Here's how the part is built. I have some questions about the finished solid (model axes, mm). Face numbers are marked on the shaded views. A direction names the side the tool comes from. Coordinates: 2 decimals unless noted, no trailing zeros. Write each loop counter-clockwise with the first axis right and the second up, starting at its lowest first coordinate (ties: lowest second). Pieces come first, ordered by that corner, then holes. Notation, with made-up numbers: M -26.5,27 L 28.5,27 A20 ccw 28.5,53 Z; hole C 65,-7.75 d5. An arc over 180 degrees is marked long. Write each question's results on one line, items separated by ' | '. Start each with the question number.
from build123d import *

# Parameters (mm, degrees)
SKETCH_1_W                     = 112
SKETCH_1_H                     = 112
SKETCH_1_W_2                   = 106
SKETCH_1_H_2                   = 106
EXTRUDE_1_DEPTH                = 45
SKETCH_3_W                     = 112
SKETCH_3_H                     = 112
EXTRUDE_2_DEPTH                = 6
SKETCH_4_R                     = 28.5
CUT_EXTRUDE_2_DEPTH            = 2
SKETCH_5_R                     = 2.05
CUT_EXTRUDE_3_DEPTH            = 3
SKETCH_6_R                     = 17
CUT_EXTRUDE_4_DEPTH            = 6
EXTRUDE_3_DEPTH                = 9
FILLET_1_R                     = 5
SKETCH_8_W                     = 85
SKETCH_8_H                     = 15
CUT_EXTRUDE_5_DEPTH            = 5
SKETCH_9_W                     = 25
SKETCH_9_H                     = 15
CUT_EXTRUDE_6_DEPTH            = 5
SKETCH_10_R                    = 2.05
CUT_EXTRUDE_7_DEPTH            = 5
FILLET_5_R                     = 5
HOLE_WIZARD_M3_5_2_D           = 3.9
HOLE_WIZARD_M3_5_2_CSINK_D     = 7.7
HOLE_WIZARD_M3_5_2_CSINK_ANGLE = 90
FILLET_START                   = 9
FILLET_7_DEPTH                 = 31
FILLET_START_2                 = 40
FILLET_7_2_DEPTH               = 5


with BuildPart() as part:
    # 草图1 → 凸台-拉伸1 (new body)
    with BuildSketch(Plane(origin=(0, 0, 0), x_dir=(1, 0, 0), z_dir=(0, 1, 0))):
        Rectangle(SKETCH_1_W, SKETCH_1_H)
        Rectangle(SKETCH_1_W_2, SKETCH_1_H_2, mode=Mode.SUBTRACT)
    extrude(amount=EXTRUDE_1_DEPTH)

    # 草图3 → 凸台-拉伸2 (add)
    with BuildSketch(Plane.XZ):
        Rectangle(SKETCH_3_W, SKETCH_3_H)
    extrude(amount=EXTRUDE_2_DEPTH)

    # 草图4 → 切除-拉伸2 (cut)
    with BuildSketch(Plane.XZ.offset(6)):
        with Locations(Location((0, 0, 0), (0, 0, 270))):
            Circle(SKETCH_4_R)
    extrude(amount=-CUT_EXTRUDE_2_DEPTH, mode=Mode.SUBTRACT)

    # 草图5 → 切除-拉伸3 (cut)
    with BuildSketch(Plane(origin=(0, -4, 0), x_dir=(-1, 0, 0), z_dir=(0, -1, 0))):
        with Locations(Location((0, -22.5, 0), (0, 0, 90))):
            Circle(SKETCH_5_R)
        with Locations(Location((-22.5, 0, 0), (0, 0, 90))):
            Circle(SKETCH_5_R)
        with Locations(Location((22.5, 0, 0), (0, 0, 90))):
            Circle(SKETCH_5_R)
        with Locations(Location((0, 22.5, 0), (0, 0, 90))):
            Circle(SKETCH_5_R)
    extrude(amount=-CUT_EXTRUDE_3_DEPTH, mode=Mode.SUBTRACT)

    # 草图6 → 切除-拉伸4 (cut)
    with BuildSketch(Plane.XZ.offset(4)):
        with Locations(Location((0, 0, 0), (0, 0, 270))):
            Circle(SKETCH_6_R)
    extrude(amount=-CUT_EXTRUDE_4_DEPTH, mode=Mode.SUBTRACT)

    # 草图7 → 凸台-拉伸3 (add)
    with BuildSketch(Plane(origin=(0, 0, 0), x_dir=(1, 0, 0), z_dir=(0, 1, 0))):
        with BuildLine():
            Line((-45, 37), (-53, 37))
            Line((-53, 37), (-53, 53))
            Line((-53, 53), (-37, 53))
            Line((-37, 53), (-37, 45))
            ThreePointArc((-37, 45), (-39.343145751, 39.343145751), (-45, 37))
        make_face()
        with BuildLine():
            Line((-45, -37), (-53, -37))
            Line((-53, -37), (-53, -53))
            Line((-53, -53), (-37, -53))
            Line((-37, -53), (-37, -45))
            ThreePointArc((-37, -45), (-39.343145751, -39.343145751), (-45, -37))
        make_face()
        with BuildLine():
            Line((45, -39), (53, -39))
            Line((53, -39), (53, -53))
            Line((53, -53), (39, -53))
            Line((39, -53), (39, -45))
            ThreePointArc((39, -45), (41, -41), (45, -39))
        make_face()
        with BuildLine():
            Line((45, 37), (53, 37))
            Line((53, 37), (53, 53))
            Line((53, 53), (37, 53))
            Line((37, 53), (37, 45))
            ThreePointArc((37, 45), (39.343145751, 39.343145751), (45, 37))
        make_face()
    extrude(amount=EXTRUDE_3_DEPTH)

    # 圆角1
    fillet_1_edges = [part.edges().sort_by_distance(p)[0] for p in [
        (56, 19.5, 56),
        (-56, 19.5, 56),
        (-56, 19.5, -56),
        (56, 19.5, -56),
    ]]
    fillet(fillet_1_edges, radius=FILLET_1_R)

    # 草图8 → 切除-拉伸5 (cut)
    with BuildSketch(Plane.ZY.offset(56)):
        with Locations((0, 34.5)):
            Rectangle(SKETCH_8_W, SKETCH_8_H)
    extrude(amount=-CUT_EXTRUDE_5_DEPTH, mode=Mode.SUBTRACT)

    # 草图9 → 切除-拉伸6 (cut)
    with BuildSketch(Plane.XY.offset(56)):
        with Locations((18.5, 34.5)):
            Rectangle(SKETCH_9_W, SKETCH_9_H)
    extrude(amount=-CUT_EXTRUDE_6_DEPTH, mode=Mode.SUBTRACT)

    # 草图10 → 切除-拉伸7 (cut)
    with BuildSketch(Plane(origin=(0, 45, 0), x_dir=(1, 0, 0), z_dir=(0, 1, 0))):
        with Locations((52.035533906, -52.035533906)):
            Circle(SKETCH_10_R)
        with Locations((-52.035533906, -52.035533906)):
            Circle(SKETCH_10_R)
        with Locations((-52.035533906, 52.035533906)):
            Circle(SKETCH_10_R)
        with Locations((52.035533906, 52.035533906)):
            Circle(SKETCH_10_R)
    extrude(amount=-CUT_EXTRUDE_7_DEPTH, mode=Mode.SUBTRACT)

    # 圆角5
    fillet_5_edges = [part.edges().sort_by_distance(p)[0] for p in [
        (56, -6, 0),
        (-56, -6, 0),
        (0, -6, -56),
        (0, -6, 56),
        (-54.535533906, -6, 54.535533906),
        (-54.535533906, -6, -54.535533906),
        (54.535533906, -6, -54.535533906),
        (54.535533906, -6, 54.535533906),
    ]]
    fillet(fillet_5_edges, radius=FILLET_5_R)

    # M3.5 十字槽半沉头木螺钉的锥形沉头孔2 (through all)
    with Locations(Plane(origin=(0, -6, 0), x_dir=(-1, 0, 0), z_dir=(0, -1, 0))):
        with Locations((0, 0), (45, -45), (-45, 45), (-45, -45), (45, 45)):
            CounterSinkHole(HOLE_WIZARD_M3_5_2_D / 2, HOLE_WIZARD_M3_5_2_CSINK_D / 2, counter_sink_angle=HOLE_WIZARD_M3_5_2_CSINK_ANGLE)

    # 圆角7: read off the stored shape, not the designer's step
    # 圆角7 outline → 圆角7 (add)
    with BuildSketch(Plane(origin=(0, 0, 0), x_dir=(1, 0, 0), z_dir=(0, 1, 0)).offset(FILLET_START)):
        with BuildLine():
            Line((53, -53), (53, -43))
            ThreePointArc((53, -43), (50.071067812, -50.071067812), (43, -53))
            Line((43, -53), (53, -53))
        make_face()
        with BuildLine():
            ThreePointArc((43, 53), (50.071067812, 50.071067812), (53, 43))
            Line((53, 43), (53, 53))
            Line((53, 53), (43, 53))
        make_face()
        with BuildLine():
            ThreePointArc((-43, -53), (-50.071067812, -50.071067812), (-53, -43))
            Line((-53, -43), (-53, -53))
            Line((-53, -53), (-43, -53))
        make_face()
        with BuildLine():
            ThreePointArc((-53, 43), (-50.071067812, 50.071067812), (-43, 53))
            Line((-43, 53), (-53, 53))
            Line((-53, 53), (-53, 43))
        make_face()
    extrude(amount=FILLET_7_DEPTH)

    # Fillet 7 2 outline → Fillet 7 2 (add)
    with BuildSketch(Plane(origin=(0, 0, 0), x_dir=(1, 0, 0), z_dir=(0, 1, 0)).offset(FILLET_START_2)):
        with BuildLine():
            ThreePointArc((50.22658251, -53), (50.585965005, -50.585965005), (53, -50.22658251))
            Line((53, -50.22658251), (53, -43))
            ThreePointArc((53, -43), (50.071067812, -50.071067812), (43, -53))
            Line((43, -53), (50.22658251, -53))
        make_face()
        with BuildLine():
            ThreePointArc((43, 53), (50.071067812, 50.071067812), (53, 43))
            Line((53, 43), (53, 50.22658251))
            ThreePointArc((53, 50.22658251), (50.585965005, 50.585965005), (50.22658251, 53))
            Line((50.22658251, 53), (43, 53))
        make_face()
        with BuildLine():
            Line((-50.22658251, -53), (-43, -53))
            ThreePointArc((-43, -53), (-50.071067812, -50.071067812), (-53, -43))
            Line((-53, -43), (-53, -50.22658251))
            ThreePointArc((-53, -50.22658251), (-50.585965005, -50.585965005), (-50.22658251, -53))
        make_face()
        with BuildLine():
            ThreePointArc((-53, 43), (-50.071067812, 50.071067812), (-43, 53))
            Line((-43, 53), (-50.22658251, 53))
            ThreePointArc((-50.22658251, 53), (-50.585965005, 50.585965005), (-53, 50.22658251))
            Line((-53, 50.22658251), (-53, 43))
        make_face()
    extrude(amount=FILLET_7_2_DEPTH)


solid = part.part
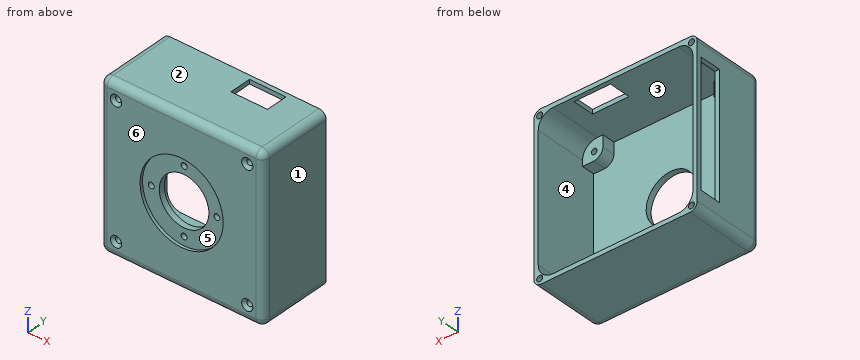
1) Please list where these lines run through material, in increasing order: line 1 (Z direction, x = 45, y = -1); line 2 (X direction, y = 3, z = -45); line 3 (Z direction, x = 45, y = 1.75). Write a range as [from, to].
2) For the marked faces 4, 5 and 6, which set-ups out of +Z, -Z, +X, -X, +Y, -Y let a thin tool reach every point of the face, with its end or its side?
3) For pin 1 Ø4.5 at (x, z) = (0, 22.5) entering from -Y; pin 2 Ø3.5 at (x, z) = (52.04, 52.04) entering from +Y; pin 3 Ø3.5 at (x, z) = (-45, 45) entering from +Y; pin 4 Ø6 at (x, z) = (45, 45) entering from -Y, each with a flat end and sliding along its axis, tell me the tip position at first contact or that it passes through.
4) I want a section at A-A, the plane x = 0. Write out the boundary of the cut face in (y, z).
5) I want a section at D-D, the plane y = 24. Write out the boundary of the cut face in (x, z), then the cut area to 3 significant figures.
6) We'd pull the mould along Z, two halves only. Please class the marked faces 1, 2 and 3: pulls with the +Z half, pulls with the -Z half, needs draft (parallel to the pull), parting line crosses it, or undercut.
7) I want a section at B-B, the plane y = 33. Write out the boundary of the cut face in (x, z), then the cut area to 3 significant figures.
8) I want a section at C-C, the plane z = 0. Give the number of separate pieces and of enclosed holes in the cut face, then the cut area to 3 significant figures.
Output:
1) line 1: z = [-56, -46.95], [-43.05, 43.05], [46.95, 56] | line 2: x = [-56, -46.95], [-43.05, -37], [37, 43.05], [46.95, 56] | line 3: z = [-56, -46.95], [-43.05, -37], [39, 43.05], [46.95, 56]
2) face 4: +Y | face 5: -Y | face 6: +Z, -Z, +X, -X, -Y
3) pin 1: stops at y = -4 | pin 2: stops at y = 40 | pin 3: passes through | pin 4: stops at y = -5.15
4) outline: M -6,-51 A5 ccw -1,-56 L 45,-56 L 45,-53 L 0,-53 L 0,-17 L -4,-17 L -4,-20.45 L -1,-20.45 L -1,-24.55 L -4,-24.55 L -4,-28.5 L -6,-28.5 Z; M -6,28.5 L -4,28.5 L -4,24.55 L -1,24.55 L -1,20.45 L -4,20.45 L -4,17 L 0,17 L 0,53 L 45,53 L 45,56 L -1,56 A5 ccw -6,51 Z
5) outline: M -56,-51 A5 ccw -51,-56 L 51,-56 A5 ccw 56,-51 L 56,51 A5 ccw 51,56 L -51,56 A5 ccw -56,51 Z; hole M -53,-43 A10 ccw -43,-53 L 43,-53 A10 ccw 53,-43 L 53,43 A10 ccw 43,53 L -43,53 A10 ccw -53,43 Z | area: 1,370 mm2
6) face 1: needs draft | face 2: pulls with the +Z half | face 3: undercut
7) outline: M -56,-51 A5 ccw -51,-56 L 51,-56 A5 ccw 56,-51 L 56,51 A5 ccw 51,56 L 31,56 L 31,53 L 43,53 A10 cw 53,43 L 53,-43 A10 cw 43,-53 L -43,-53 A10 cw -53,-43 L -53,-42.5 L -56,-42.5 Z; M -56,42.5 L -53,42.5 L -53,43 A10 cw -43,53 L 6,53 L 6,56 L -51,56 A5 ccw -56,51 Z | area: 1,040 mm2
8) separate pieces: 3 | enclosed holes: 0 | area: 612 mm2
